Autodesk Inventor part; units mm, degrees
ref_plane "YZ Plane" through (0, 0, 0) normal (1, 0, 0) x (0, 1, 0)
ref_plane "XZ Plane" through (0, 0, 0) normal (0, 1, 0) x (-1, 0, 0)
ref_plane "XY Plane" through (0, 0, 0) normal (0, 0, 1) x (1, 0, 0)
sketch "スケッチ1" plane through (0, 0, 0) normal (0, 1, 0) x (-1, 0, 0)
  line L0 (0, 0) -> (0, -24) construction
  circle A0 centre (0, -24) radius 4
  arc A1 (-9.3528, -20.4608) -> (9.3528, -20.4608) centre (0, -24) ccw
  line L1 (11, -2) -> (-11, -2) construction
  line L2 (-11, -2) -> (-11, 2)
  line L3 (11, 2) -> (11, -2)
  line L4 (11, 0) -> (-11, 0) construction
  circle A2 centre (8, 0) radius 1.05
  circle A3 centre (-8, 0) radius 1.05
  circle A4 centre (0, -24) radius 8 construction
  circle A5 centre (5.6569, -18.3431) radius 1.05
  circle A6 centre (0, -16) radius 1.05
  circle A7 centre (-5.6569, -18.3431) radius 1.05
  circle A8 centre (-8, -24) radius 1.05
  circle A9 centre (-5.6569, -29.6569) radius 1.05
  circle A10 centre (0, -32) radius 1.05
  circle A11 centre (5.6569, -29.6569) radius 1.05
  circle A12 centre (8, -24) radius 1.05
  line L5 (-3.05, 2) -> (-3.05, -0.9893)
  line L6 (-3.05, -2.05) -> (-1.9893, -2.05) construction
  arc A13 (1.9893, -2.05) -> (3.05, -0.9893) centre (2.5197, -1.5197) ccw
  line L7 (3.05, -2.05) -> (2.5197, -1.5197) construction
  line L8 (3.05, -0.9893) -> (3.05, 2)
  arc A14 (-3.05, -0.9893) -> (-1.9893, -2.05) centre (-2.5197, -1.5197) ccw
  line L9 (-3.05, -2.05) -> (-2.5197, -1.5197) construction
  line L10 (-3.05, -0.9893) -> (-3.05, -2.05) construction
  line L11 (-1.9893, -2.05) -> (1.9893, -2.05)
  line L12 (3.05, -0.9893) -> (3.05, -2.05) construction
  line L13 (1.9893, -2.05) -> (3.05, -2.05) construction
  line L14 (-11, 2) -> (-3.05, 2)
  line L15 (3.05, 2) -> (11, 2)
  arc A15 (10.863, -2.5052) -> (11, -2) centre (10, -2) ccw
  arc A16 (10.863, -2.5052) -> (9.3528, -20.4608) centre (28.9008, -13.0637) ccw
  line L16 (8, -6.3971) -> (8, -16.9723) construction
  arc A17 (-11, -2) -> (-10.863, -2.5052) centre (-10, -2) ccw
  arc A18 (-9.3528, -20.4608) -> (-10.863, -2.5052) centre (-28.9008, -13.0637) ccw
  dimension "d18" = 16
  dimension "d0" = 22
  dimension "d1" = 8
  dimension "d2" = 10
  dimension "d5" = 16
  dimension "d6" = 2.1
  dimension "d16" = 360
  dimension "d19" = 2.1
  dimension "d20" = 22
  dimension "d23" = 0.75
  dimension "d26" = 6.1
  dimension "d28" = 45
  dimension "d29" = 0.75
  dimension "d30" = 45
  dimension "d32" = 4
  dimension "d33" = 4.05
  dimension "d34" = 1
  dimension "d35" = 16
extrude "押し出し1" add sketch "スケッチ1" along normal blind 2
chamfer "面取り1" distance 0.25 angle 45 4 edges at (11, 1, 2) (-11, 1, 2) (-3.05, 1, 2) (3.05, 1, 2)
sketch "Sketch6" plane through (0, 2, 0) normal (0, 1, 0) x (1, 0, 0)
  line L0 (3.3, -2) -> (3.05, -1.75)
  line L1 (3.3, -2) -> (10.75, -2)
  line L2 (11, -1.75) -> (10.75, -2)
  line L3 (11, -1.75) -> (11, 2)
  arc A0 (11, 2) -> (10.863, 2.5052) centre (10, 2) ccw
  arc A1 (9.3528, 20.4608) -> (10.863, 2.5052) centre (28.9008, 13.0637) ccw
  arc A2 (9.3528, 20.4608) -> (-9.3528, 20.4608) centre (0, 24) ccw
  arc A3 (-10.863, 2.5052) -> (-9.3528, 20.4608) centre (-28.9008, 13.0637) ccw
  arc A4 (-10.863, 2.5052) -> (-11, 2) centre (-10, 2) ccw
  line L4 (-11, 2) -> (-11, -1.75)
  line L5 (-10.75, -2) -> (-11, -1.75)
  line L6 (-10.75, -2) -> (-3.3, -2)
  line L7 (-3.05, -1.75) -> (-3.3, -2)
  line L8 (-3.05, -1.75) -> (-3.05, 0.9893)
  arc A5 (-1.9893, 2.05) -> (-3.05, 0.9893) centre (-2.5197, 1.5197) ccw
  line L9 (-1.9893, 2.05) -> (1.9893, 2.05)
  arc A6 (3.05, 0.9893) -> (1.9893, 2.05) centre (2.5197, 1.5197) ccw
  line L10 (3.05, 0.9893) -> (3.05, -1.75)
  circle A7 centre (0, 24) radius 4
  circle A8 centre (-8, 24) radius 1.05
  circle A9 centre (-5.6569, 29.6569) radius 1.05
  circle A10 centre (0, 32) radius 1.05
  circle A11 centre (5.6569, 29.6569) radius 1.05
  circle A12 centre (8, 24) radius 1.05
  circle A13 centre (5.6569, 18.3431) radius 1.05
  circle A14 centre (0, 16) radius 1.05
  circle A15 centre (-5.6569, 18.3431) radius 1.05
  circle A16 centre (8, 0) radius 1.05
  circle A17 centre (-8, 0) radius 1.05
  point P0 (0, 0)
properties part number "16_046_COXA_FRAME_5_R1"
The listing builds one solid part. Answer for the finished solid, in the listing's coordinates (mm). A direction names the side the tool comes from. Give positions to 0.01 mm unless a question says otherwise; leave off trailing zeros. Loops run counter-clockwise (first coordinate to the right, second up) from the corner with the lowest first, then second, coordinate; pieces in that order, holes last. Notation, with made-up numbers: (-32, 18) - (2, 18) arc R22 cw to (2, 25) - close; hole circle Ø7 at (40, 9.25). An arc over 180 degrees is marked (long way). Return JSON: item names as keys, results as strings. Group by question number.
1. Find section B-B (x = 0). Write down the section's boundary in (y, z), then the cut area to 3 significant figures.
2. Find section C-C (z = -32). Write down the section's boundary in (x, y), then the cut area to 3 significant figures.
3. Find section A-A (z = 0). Write down the section's boundary in (x, y), then the cut area to 3 significant figures.
4. Determine the mould class of faces 3 (the flat face through (0, 1, -2.05)), 4 (the flat face through (-2, 0, -16)), 5 (the cylindrical face through (5.794, 0.986, -19.384)) for opening direction Z: pulls with the +Z half, pulls with the -Z half, needs draft (parallel to the pull), parting line crosses it, or undercut.
5. Straight lines are drawn through the part: line 1 (X direction, y = 1.85, z = -1.5); line 2 (X direction, y = 1.8, z = -24.5); line 3 (Z direction, x = 0, y = 1.35). For each, find the intervals that lie inside material, in ascending order. Write a range as [from, to].
6. Find section D-D (y = 1.2). State how many separate pieces and enclosed holes the cut face has, then the cut area to 3 significant figures.
7. Which of the six approach directions +Z, -Z, +X, -X, +Y, -Y give full straight-line access (tool end or side, diameter ignored) to faces 1 (the flat face through (3.05, 1, 0)), 2 (the cylindrical face through (9.05, 0.99, -0.05))?
8. Given pin 1 Ø1.7 at (x, z) = (-5.66, -29.66) entering from -Y; pin 2 Ø1 at (y, z) = (1, -26) entering from -X; pin 3 Ø0.6 at (x, y) = (-0.5, 0.5) entering from +Z, each flat-ended and moving along its own axis, determine where each tip first touches the part or whether it passes through.
Verdict:
{
 "1": {"outline": "(0, -34) - (2, -34) - (2, -33.05) - (0, -33.05) - close; (0, -30.95) - (2, -30.95) - (2, -28) - (0, -28) - close; (0, -20) - (2, -20) - (2, -17.05) - (0, -17.05) - close; (0, -14.95) - (2, -14.95) - (2, -2.05) - (0, -2.05) - close", "area": "39.5 mm^2"},
 "2": {"outline": "(-6, 0) - (-1.05, 0) - (-1.05, 2) - (-6, 2) - close; (1.05, 0) - (6, 0) - (6, 2) - (1.05, 2) - close", "area": "19.8 mm^2"},
 "3": {"outline": "(-11, 0) - (-9.05, 0) - (-9.05, 2) - (-11, 2) - close; (-6.95, 0) - (-3.05, 0) - (-3.05, 2) - (-6.95, 2) - close; (3.05, 0) - (6.95, 0) - (6.95, 2) - (3.05, 2) - close; (9.05, 0) - (11, 0) - (11, 2) - (9.05, 2) - close", "area": "23.4 mm^2"},
 "4": {"face 3": "pulls with the +Z half", "face 4": "needs draft", "face 5": "undercut"},
 "5": {"line 1": "x = [-11, -3.27], [3.27, 11]", "line 2": "x = [-9.99, -8.92], [-7.08, -3.97], [3.97, 7.08], [8.92, 9.99]", "line 3": "z = [-34, -33.05], [-30.95, -28], [-20, -17.05], [-14.95, -2.05]"},
 "6": {"separate pieces": "1", "enclosed holes": "11", "area": "528 mm^2"},
 "7": {"face 1": "+Z, +Y, -Y", "face 2": "+Y, -Y"},
 "8": {"pin 1": "passes through", "pin 2": "stops at x = -9.89", "pin 3": "stops at z = -2.05"}
}
